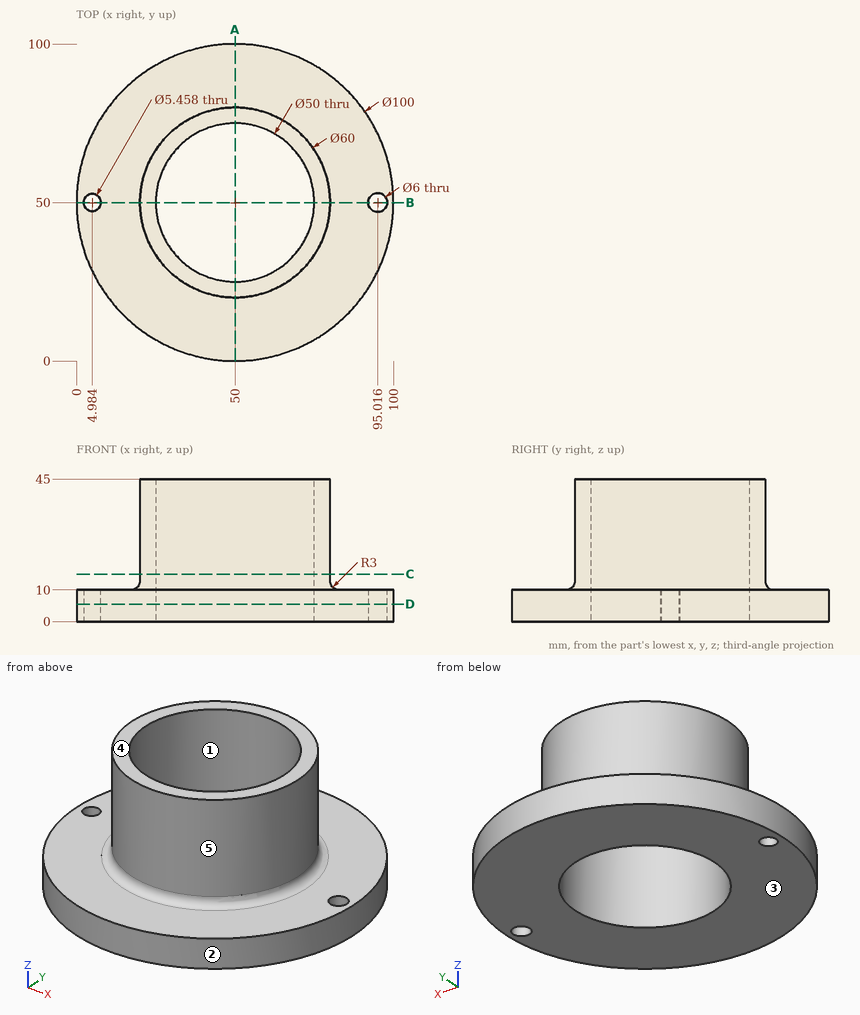
Design review of the part shown in the three views and the two pictorial views. Dimensions are in mm from the part's minimum x, y and z. A direction names the side the tool comes from. Give positions to 0.01 mm unless a question says otherwise; leave off trailing zeros. Loops run counter-clockwise (first coordinate to the right, second up) from the corner with the lowest first, then second, coordinate; pieces in that order, holes last. Notation, with made-up numbers: (-3.5, 89.25) -> (40.5, 89.25) arc R14 ccw to (40.5, 96.25) -> close; hole circle Ø3 at (49.25, 25.25). An arc over 180 degrees is marked (long way). Put each result on its own line as item: value. Start each with the question number.
1. Mouldability with a two-part tool opening along X and no side actions: class the marked faces 1, 2 and 3 as released by +X, released by -X, zero draft, split by the parting line, or undercut.
2. Clearance check with flat-ended pins moving along their axes: P1, Ø1.5, axis at x = 45, z = 29, coming from the -Y side; P2, Ø12, axis at x = 86, z = 6.5, coming from the -Y side; P3, Ø8, axis at y = 76.5, z = 9, coming from the +X side; P4, Ø5, axis at x = 95.02, y = 50, coming from the +Z side. State where each tip first meets the part, or that it passes through.
3. Wall thickness on probe 1 along Y at (x, z) = (50, 21); probe 2 along Z at (x, y) = (74.5, 85); probe 3 along Y at (x, z) = (73, 13) (1 decimal): over which ranges is each line inside the solid? List them lowest first.
4. For the marked faces 4 and 5, list the 3-axis set-ups (+Z, -Z, +X, -X, +Y, -Y) from which the entire face can be reached by the end or side of a thin tool; tool diameter is ignored.
5. We need section B-B on y = 50. State the section outline as (x, z) points (1 decimal).
6. We need section A-A on x = 50. State the section outline as (y, z) points, then the cut area to 3 significant figures.
7. We need section D-D on z = 5.5. State the section outline as (x, y) points.
8. We need section C-C on z = 15. State the section outline as (x, y) points, then the cut area to 3 significant figures.
Determined:
1. face 1: undercut
1. face 2: split by the parting line
1. face 3: zero draft
2. P1: y = 20.3
2. P2: y = 10
2. P3: x = 94.65
2. P4: through
3. probe 1: 20 to 25, 75 to 80
3. probe 2: 0 to 10
3. probe 3: 30.7 to 40.2, 59.8 to 69.3
4. face 4: +Z, +X, -X, +Y, -Y
4. face 5: +Z
5. outline: (0, 0) -> (2.3, 0) -> (2.3, 10) -> (0, 10) -> close; (7.7, 0) -> (25, 0) -> (25, 45) -> (20, 45) -> (20, 13) arc R3 cw to (17, 10) -> (7.7, 10) -> close; (75, 0) -> (92, 0) -> (92, 10) -> (83, 10) arc R3 cw to (80, 13) -> (80, 45) -> (75, 45) -> close; (98, 0) -> (100, 0) -> (100, 10) -> (98, 10) -> close
6. outline: (0, 0) -> (25, 0) -> (25, 45) -> (20, 45) -> (20, 13) arc R3 cw to (17, 10) -> (0, 10) -> close; (75, 0) -> (100, 0) -> (100, 10) -> (83, 10) arc R3 cw to (80, 13) -> (80, 45) -> (75, 45) -> close
6. area: 854 mm^2
7. outline: circle Ø100 at (50, 50); hole circle Ø5.46 at (4.98, 50); hole circle Ø50 at (50, 50); hole circle Ø6 at (95.02, 50)
8. outline: circle Ø60 at (50, 50); hole circle Ø50 at (50, 50)
8. area: 864 mm^2
